Can you work these out from the model? Positions are in its coordinate system, mm. Round coordinates to 2 decimals unless told otherwise and drop trailing zeros. Loops run counter-clockwise (first coordinate to the right, second up) from the corner with the lowest first, then second, coordinate; pieces in that order, holes last. Notation, with made-up numbers: M 89,-16 L 103,-16 A36 ccw 103,21 Z; hole C 56,23 d3. An arc over 180 degrees is marked long. Return JSON: item names as keys, results as strings.
```python
from build123d import *

# Parameters (mm, degrees)
ESQUISSE1_R        = 14.5
BOSS_EXTRU_1_DEPTH = 13
ESQUISSE2_R        = 0.190045057
BOSS_EXTRU_2_DEPTH = 6


with BuildPart() as part:
    # Esquisse1 → Boss.-Extru.1 (new body)
    with BuildSketch(Plane(origin=(0, 0, 0), x_dir=(1, 0, 0), z_dir=(0, 1, 0))):
        with Locations(Location((0, 0, 0), (0, 0, 90))):
            Circle(ESQUISSE1_R)
    extrude(amount=BOSS_EXTRU_1_DEPTH)

    # Esquisse2 → Boss.-Extru.2 (add)
    with BuildSketch(Plane(origin=(0, 13, 0), x_dir=(1, 0, 0), z_dir=(0, 1, 0))):
        with Locations(Location((-6.864876716, 0, 0), (0, 0, 270))):
            Circle(ESQUISSE2_R)
    boss_extru_2 = extrude(amount=BOSS_EXTRU_2_DEPTH)

    # Symétrie1: Boss.-Extru.2 across plane
    add(boss_extru_2.mirror(Plane(origin=(0, 0, 0), x_dir=(0, 0, 1), z_dir=(1, 0, 0))))


solid = part.part
```
Q1. Suppose I cut it at C-C, the plane y = 4.75. Please give me the cut outline in (x, z).
Results:
{"outline": "C 0,0 d29"}
Q2. Suppose I cut it at A-A, the plane z = 10.5. Please give me the cut outline in (x, y).
Results:
{"outline": "M -10,0 L 10,0 L 10,13 L -10,13 Z"}
Q3. If I drill on line 1 along Y through (x, z) = (7, -3.25); line 2 along X through (y, z) = (9.5, -0.25); line 3 along X through (y, z) = (6, -11.5), over which ranges is the centre line in solid material (lowest first)?
Results:
{"line 1": "y = 0 to 13", "line 2": "x = -14.5 to 14.5", "line 3": "x = -8.83 to 8.83"}
Q4. I'm going to push flat-ended pins straight in: pin 1 Ø3 at (x, z) = (7, 5.5) entering from +Y; pin 2 Ø1 at (y, z) = (12.5, 1.5) entering from -X; pin 3 Ø2 at (y, z) = (8, 3.5) entering from -X. Where does each tip first touch, or does it pass through?
Results:
{"pin 1": "stops at y = 13", "pin 2": "stops at x = -14.47", "pin 3": "stops at x = -14.28"}
Q5. Suppose I cut it at D-D, the plane y = 13.75. Please give me the cut outline in (x, z).
Results:
{"outline": "C -6.86,0 d0.38; C 6.86,0 d0.38"}
Q6. Suppose I cut it at B-B, the plane x = 0. Please give me the cut outline in (y, z), plus the area to 3 significant figures.
Results:
{"outline": "M 0,-14.5 L 13,-14.5 L 13,14.5 L 0,14.5 Z", "area": "377 mm2"}
